Could you check a few things on this model? Use its own coordinates, in mm. A direction names the side the tool comes from. Give positions to 0.01 mm unless a question says otherwise; leave off trailing zeros. Loops run counter-clockwise (first coordinate to the right, second up) from the corner with the lowest first, then second, coordinate; pieces in that order, holes last. Notation, with made-up numbers: M -28,-22 L 9,-22 A25 cw 9,9 Z; hole C 24.25,88.25 d1. An arc over 180 degrees is marked long. Return JSON: item names as keys, results as strings. Group by question number.
1. For pin 1 (1.5 mm diameter, centred on x = 3, z = -3, fed in from -Y); pin 2 (1 mm diameter, centred on x = -2.5, z = -3, fed in from +Y); pin 3 (1.6 mm diameter, centred on x = -5, y = -1, fed in from +Z) (3 decimals), each with a flat end and sliding along its axis, tell me the tip position at first contact or that it passes through.
2. If we section it at C-C (x = -4): Write out the boundary of the cut face in (y, z), plus the area to 3 significant figures.
3. If we mould it in two halves opening along X, with no side actions, what happens to faces 1 (the conical face through (-5.8, -0.1, -3.6)), 2 (the cylindrical face through (-0.766, -0.056, 1.847)), 3 (the flat face through (-5, 0, 0.75))? For each: +X half, -X half, draft (parallel to the pull), parting line (faces both ways), or undercut.
4. If we section it at A-A (z = 0): Write out the boundary of the cut face in (x, y).
5. Please list where these lines run through material, in increasing order: line 1 (Z direction, x = 0, y = 0); line 2 (X direction, y = -1.75, z = -0.25); line 3 (X direction, y = -2, z = 0.5).
6. For faces 4 (the flat face through (6, 0, 0)), 5 (the flat face through (-5, 0, -0.75)), which set-ups out of +Z, -Z, +X, -X, +Y, -Y let a thin tool reach every point of the face, with its end or its side?
7. If we section it at D-D (x = -0.75): Write out the boundary of the cut face in (y, z).
8. If we section it at B-B (y = 0): Write out the boundary of the cut face in (x, z), plus the area to 3 significant figures.
```python
from build123d import *

# Parameters (mm, degrees)
SKETCH1_R               = 4
BOSS_EXTRUDE1_DEPTH     = 6
CHAMFER1_SIZE           = 0.6
CUT_EXTRUDE1_DEPTH      = 9.246211251
CUT_EXTRUDE1_DEPTH_BACK = 9.246211251
SKETCH2_R               = 2
SKETCH3_W               = 1.5
SKETCH3_H               = 10.178727068
CUT_EXTRUDE2_DEPTH      = 1.5


with BuildPart() as part:
    # Sketch1 → Boss-Extrude1 (new, symmetric)
    with BuildSketch(Plane(origin=(0, 0, 0), x_dir=(0, 0, -1), z_dir=(1, 0, 0))):
        Circle(SKETCH1_R)
    extrude(amount=BOSS_EXTRUDE1_DEPTH, both=True)

    # Chamfer1
    chamfer1_edges = [part.edges().sort_by_distance(p)[0] for p in [
        (-6, 0, 4),
        (6, 0, 4),
    ]]
    chamfer(chamfer1_edges, length=CHAMFER1_SIZE)

    # Sketch2 → Cut-Extrude1 (cut, two sides: drawn at the far end of the back side and taken through both)
    with BuildSketch(Plane(origin=(0, 0, 0), x_dir=(1, 0, 0), z_dir=(0, 1, 0)).offset(-CUT_EXTRUDE1_DEPTH_BACK)):
        with Locations(Location((0, 0, 0), (0, 0, 270))):
            Circle(SKETCH2_R)
    extrude(amount=CUT_EXTRUDE1_DEPTH + CUT_EXTRUDE1_DEPTH_BACK, mode=Mode.SUBTRACT)

    # Sketch3 → Cut-Extrude2 (cut)
    with BuildSketch(Plane.ZY.offset(6)):
        Rectangle(SKETCH3_W, SKETCH3_H)
    extrude(amount=-CUT_EXTRUDE2_DEPTH, mode=Mode.SUBTRACT)


solid = part.part
```
Answer:
{
 "1": {"pin 1": "stops at y = -3.31", "pin 2": "stops at y = 3.12", "pin 3": "stops at z = 3.995"},
 "2": {"outline": "C 0,0 d8", "area": "50.3 mm²"},
 "3": {"face 1": "-X half", "face 2": "undercut", "face 3": "draft"},
 "4": {"outline": "M -4.5,-4 L -2,-4 L -2,4 L -4.5,4 Z; M 2,-4 L 5.4,-4 L 6,-3.4 L 6,3.4 L 5.4,4 L 2,4 Z"},
 "5": {"line 1": "z = -4 to -2, 2 to 4", "line 2": "x = -4.5 to -1.98, 1.98 to 6", "line 3": "x = -4.5 to -1.94, 1.94 to 6"},
 "6": {"face 4": "+Z, -Z, +X, +Y, -Y", "face 5": "-X, +Y, -Y"},
 "7": {"outline": "M -3.54,-1.85 A4 ccw 3.54,-1.85 Z; M -3.54,1.85 L 3.54,1.85 A4 ccw Z"},
 "8": {"outline": "M -6,-3.4 L -5.4,-4 L 5.4,-4 L 6,-3.4 L 6,3.4 L 5.4,4 L -5.4,4 L -6,3.4 L -6,0.75 L -4.5,0.75 L -4.5,-0.75 L -6,-0.75 Z; hole C 0,0 d4", "area": "80.5 mm²"}
}
